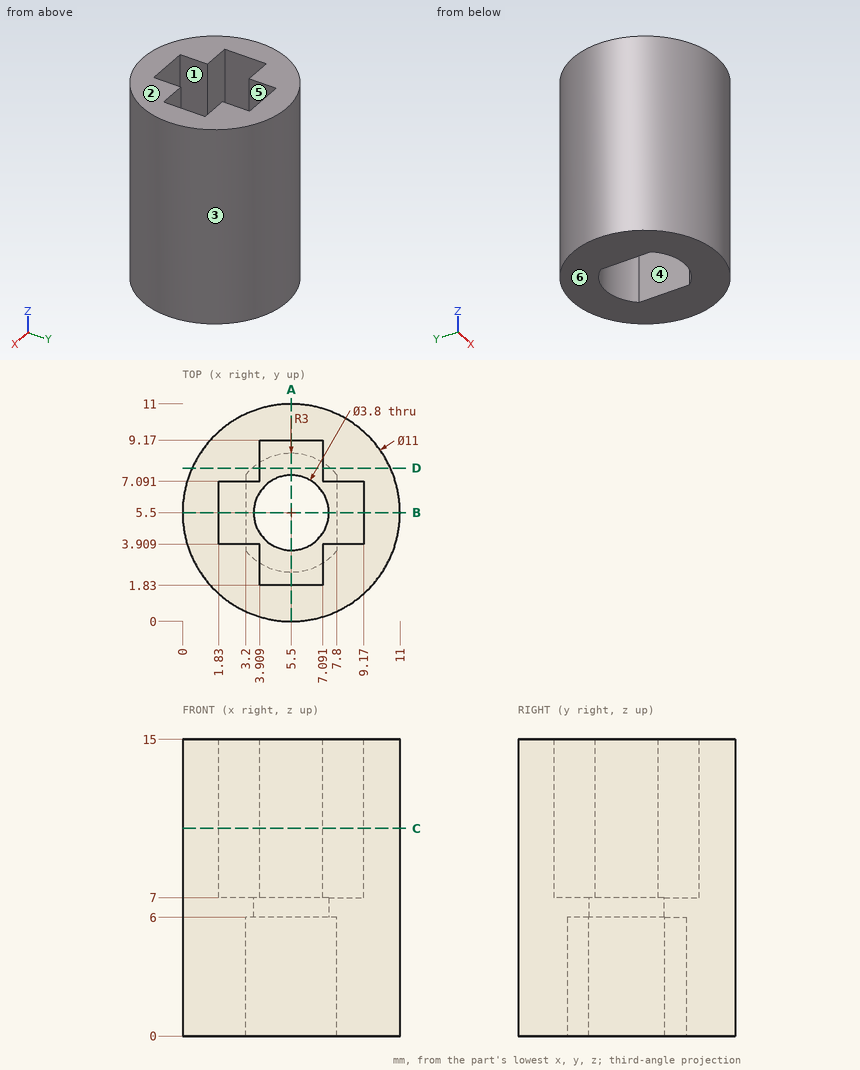
For this review, use the dimensioned drawing (mm, ordinates from the lowest corner) and the shaded views. A direction names the side the tool comes from. Round coordinates to 2 decimals unless told otherwise and drop trailing zeros. Loops run counter-clockwise (first coordinate to the right, second up) from the corner with the lowest first, then second, coordinate; pieces in that order, holes last. Notation, with made-up numbers: M 43,47 L 56,47 A10 ccw 56,53 Z; hole C -11,86.25 d3. An arc over 180 degrees is marked long. Answer as CSV lines item,"result".
1. Insertion check: pin 1 Ø3 at (y, z) = (5, 2) entering from +X; pin 2 Ø0.6 at (y, z) = (8.5, 11) entering from +X; pin 3 Ø2.5 at (y, z) = (3.5, 12.5) entering from +X; pin 4 Ø0.6 at (y, z) = (8, 9.5) entering from -X. Each pin has a flat end and moves straight along its axis. Give the tip position at first contact, or say it passes through.
Outcome:
pin 1,"stops at x = 11"
pin 2,"stops at x = 10.29"
pin 3,"stops at x = 10.95"
pin 4,"stops at x = 0.46"
2. We need section A-A (x = 5.5). Give the boundary of the cut face in (y, z).
Outcome:
outline,"M 0,0 L 2.5,0 L 2.5,6 L 3.6,6 L 3.6,7 L 1.83,7 L 1.83,15 L 0,15 Z; M 7.4,6 L 8.5,6 L 8.5,0 L 11,0 L 11,15 L 9.17,15 L 9.17,7 L 7.4,7 Z"
3. Draft analysis for pull direction Y (two halves, no side actions). For the marked faces 1, 2 and 3, state which applies: pulls with the +Y half, pulls with the -Y half, needs draft (parallel to the pull), parting line crosses it, or undercut.
Outcome:
face 1,"undercut"
face 2,"needs draft"
face 3,"parting line crosses it"
4. To check wall thickness, follow L1, parallel to Y at x = 5.5, z = 6.35; L2, parallel to X at y = 7.75, z = 4; L3, parallel to X at y = 6, z = 5.25. State the ranges of each line that lie inside material, in increasing order. Write a range as [from, to].
Outcome:
L1,"y = [0, 3.6], [7.4, 11]"
L2,"x = [0.48, 3.52], [7.48, 10.52]"
L3,"x = [0.02, 3.2], [7.8, 10.98]"
5. We need section B-B (y = 5.5). Give the boundary of the cut face in (x, z).
Outcome:
outline,"M 0,0 L 3.2,0 L 3.2,6 L 3.6,6 L 3.6,7 L 1.83,7 L 1.83,15 L 0,15 Z; M 7.4,6 L 7.8,6 L 7.8,0 L 11,0 L 11,15 L 9.17,15 L 9.17,7 L 7.4,7 Z"
6. For the marked faces 4, 5 and 6, list the 3-axis set-ups (+Z, -Z, +X, -X, +Y, -Y) from which the entire face can be reached by the end or side of a thin tool; tool diameter is ignored.
Outcome:
face 4,"-Z"
face 5,"+Z"
face 6,"-Z, +X, -X, +Y, -Y"
7. We need section D-D (y = 7.75). Give the boundary of the cut face in (x, z), plus the area to 3 significant figures.
Outcome:
outline,"M 0.48,0 L 3.52,0 L 3.52,6 L 7.48,6 L 7.48,0 L 10.52,0 L 10.52,15 L 7.09,15 L 7.09,7 L 3.91,7 L 3.91,15 L 0.48,15 Z"
area,"101 mm2"
8. We need section C-C (z = 10.5). Give the boundary of the cut face in (x, y), plus the area to 3 significant figures.
Outcome:
outline,"C 5.5,5.5 d11; hole M 1.83,3.91 L 3.91,3.91 L 3.91,1.83 L 7.09,1.83 L 7.09,3.91 L 9.17,3.91 L 9.17,7.09 L 7.09,7.09 L 7.09,9.17 L 3.91,9.17 L 3.91,7.09 L 1.83,7.09 Z"
area,"58.4 mm2"
